Verification items for the finished model (mm, model axes). Face numbers are marked on the shaded views. Round coordinates to 2 decimals unless told otherwise and drop trailing zeros. Write each loop counter-clockwise with the first axis right and the second up, starting at its lowest first coordinate (ties: lowest second). Pieces come first, ordered by that corner, then holes. Notation, with made-up numbers: (20.5, -31) - (70.5, -31) arc R14 ccw to (70.5, -18) - close; hole circle Ø11 at (51.25, 71). An arc over 180 degrees is marked (long way). Answer as a JSON object with one key per item and string values.
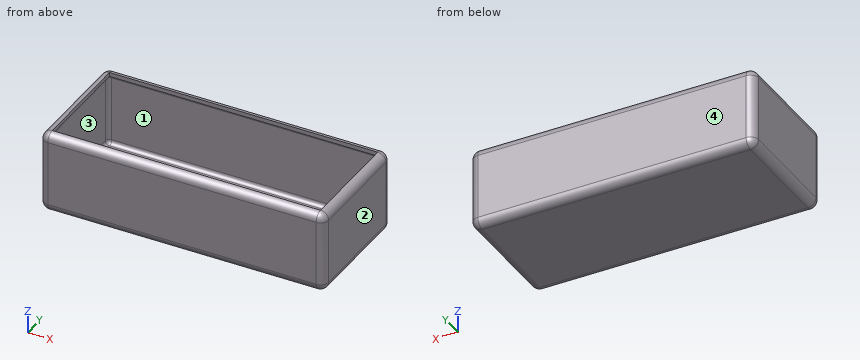
```python
from build123d import *

# Parameters (mm, degrees)
F0_W     = 177.8
F0_H     = 50.8
F1_DEPTH = 76.2
F2_R     = 5.08
F3_T     = -2.54


# Not quite as in the source:
# - a shell that OpenCascade refuses in one call is made with other operations: the cavity is built on its own and cut out


with BuildPart() as f1:
    # F0 (on Front) → F1 (new body)
    with BuildSketch(Plane.XZ):
        with Locations((88.9, 25.4)):
            Rectangle(F0_W, F0_H)
    extrude(amount=F1_DEPTH)

    # F2
    f2_edges = [f1.edges().sort_by_distance(p)[0] for p in [
        (88.9, -76.2, 50.8),
        (177.8, -38.1, 50.8),
        (177.8, -76.2, 25.4),
        (88.9, -76.2, 0),
        (177.8, -38.1, 0),
        (177.8, 0, 25.4),
        (88.9, 0, 50.8),
        (0, 0, 25.4),
        (88.9, 0, 0),
        (0, -38.1, 50.8),
        (0, -38.1, 0),
        (0, -76.2, 25.4),
    ]]
    fillet(f2_edges, radius=F2_R)

    # F3: a shell. OpenCascade refuses it in one call, so the cavity is built on its own and cut out:
    # the body offset inwards by the wall thickness, plus a prism from it out through each open face.
    f3_core = offset(f1.part, amount=F3_T, mode=Mode.PRIVATE)
    f3_exits = [f3_core.faces().sort_by_distance(p)[0] for p in [
        (88.9, -38.1, 48.26),
    ]]
    add(f3_core, mode=Mode.SUBTRACT)
    extrude(f3_exits, amount=-F3_T, mode=Mode.SUBTRACT)


solid = f1.part
```
Q1. Gauge pin test, flat ends, axial feed: P1, Ø0.8, axis at y = -27, z = 49.5, coming from the -X side; P2, Ø2, axis at x = 83, z = 49, coming from the +Y side; P3, Ø10, axis at x = 132, y = -48.5, coming from the +Z side; P4, Ø10, axis at y = -40.5, z = 28.5, coming from the -X side. Record the tip position at first contact, or that the pin passes through.
Geometry check:
{"P1": "stops at x = 1.29", "P2": "stops at y = -0.54", "P3": "stops at z = 2.54", "P4": "stops at x = 0"}
Q2. Section check C-C, the plane y = -52.5. Record the cut outline in (x, z).
Geometry check:
{"outline": "(0, 5.08) arc R5.08 ccw to (5.08, 0) - (172.72, 0) arc R5.08 ccw to (177.8, 5.08) - (177.8, 45.72) arc R5.08 ccw to (172.72, 50.8) - (172.72, 48.26) arc R2.54 cw to (175.26, 45.72) - (175.26, 5.08) arc R2.54 cw to (172.72, 2.54) - (5.08, 2.54) arc R2.54 cw to (2.54, 5.08) - (2.54, 45.72) arc R2.54 cw to (5.08, 48.26) - (5.08, 50.8) arc R5.08 ccw to (0, 45.72) - close"}
Q3. Material ranges on line 1 along X through (y, z) = (-54.5, 15.5); line 2 along Y through (x, z) = (161.5, 36); line 3 along Z through (x, y) = (71, -5), recorded low to high. Write a range as [from, to].
Geometry check:
{"line 1": "x = [0, 2.54], [175.26, 177.8]", "line 2": "y = [-76.2, -73.66], [-2.54, 0]", "line 3": "z = [0, 2.54], [48.26, 50.8]"}
Q4. Section check B-B, the plane x = 82. Record the cut outline in (y, z).
Geometry check:
{"outline": "(-76.2, 5.08) arc R5.08 ccw to (-71.12, 0) - (-5.08, 0) arc R5.08 ccw to (0, 5.08) - (0, 45.72) arc R5.08 ccw to (-5.08, 50.8) - (-5.08, 48.26) arc R2.54 cw to (-2.54, 45.72) - (-2.54, 5.08) arc R2.54 cw to (-5.08, 2.54) - (-71.12, 2.54) arc R2.54 cw to (-73.66, 5.08) - (-73.66, 45.72) arc R2.54 cw to (-71.12, 48.26) - (-71.12, 50.8) arc R5.08 ccw to (-76.2, 45.72) - close"}
Q5. Section check A-A, the plane z = 24. Record the cut outline in (x, y), then the cut area to 3 significant figures.
Geometry check:
{"outline": "(0, -71.12) arc R5.08 ccw to (5.08, -76.2) - (172.72, -76.2) arc R5.08 ccw to (177.8, -71.12) - (177.8, -5.08) arc R5.08 ccw to (172.72, 0) - (5.08, 0) arc R5.08 ccw to (0, -5.08) - close; hole (2.54, -71.12) arc R2.54 ccw to (5.08, -73.66) - (172.72, -73.66) arc R2.54 ccw to (175.26, -71.12) - (175.26, -5.08) arc R2.54 ccw to (172.72, -2.54) - (5.08, -2.54) arc R2.54 ccw to (2.54, -5.08) - close", "area": "1,250 mm2"}
Q6. Release check for a two-part mould opening along Y. For the marked faces 1, 2, 3 and 4 record: released by +Y, released by -Y, zero draft, split by the parting line, or undercut.
Geometry check:
{"face 1": "undercut", "face 2": "zero draft", "face 3": "undercut", "face 4": "released by +Y"}
